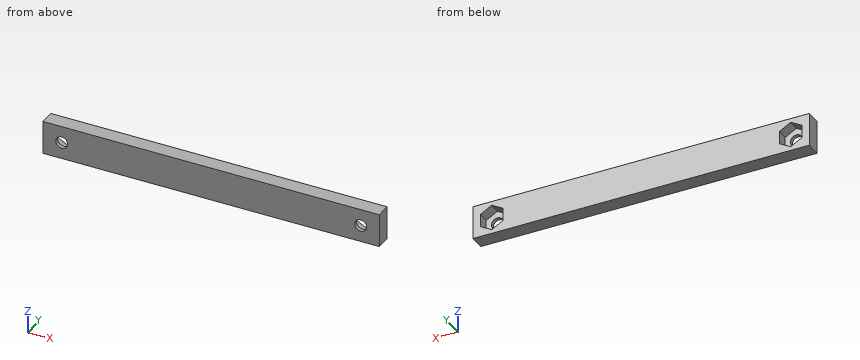
from build123d import *

# Parameters (mm, degrees)
SKETCH089_W     = 90
SKETCH089_H     = 9
SKETCH089_R     = 1.6
PAD034_DEPTH    = 4
POCKET055_DEPTH = 3


with BuildPart() as part:
    # Sketch089 → Pad034 (new body)
    with BuildSketch(Plane.XZ):
        with Locations((0, 34)):
            Rectangle(SKETCH089_W, SKETCH089_H)
        with Locations((-40, 34)):
            Circle(SKETCH089_R, mode=Mode.SUBTRACT)
        with Locations((40, 34)):
            Circle(SKETCH089_R, mode=Mode.SUBTRACT)
    extrude(amount=PAD034_DEPTH)

    # Sketch090 (on Face7 of Pad034) → Pocket055 (cut)
    with BuildSketch(Plane(origin=(0, 0, 0), x_dir=(1, 0, 0), z_dir=(0, 1, 0))):
        Polygon((-37, -32.267949), (-40, -30.535898), (-43, -32.267949), (-43, -35.732051), (-40, -37.464102), (-37, -35.732051), align=None)
    pocket055 = extrude(amount=-POCKET055_DEPTH, mode=Mode.SUBTRACT)

    # Mirrored005: Pocket055 across Sketch090 V_Axis
    add(pocket055.mirror(Plane.YZ), mode=Mode.SUBTRACT)


with BuildPart() as part_1:
    # Body012 placement: moved
    add(part.part.moved(Location((0, 19, 100))))


solid = part_1.part
The listing builds one solid part. Answer for the finished solid, in the listing's coordinates (mm). Coordinates: 2 decimals unless noted, no trailing zeros. Order: outer loops, then holes, each group sorted by start corner. A loop starts at its lowest first (then second) coordinate and runs counter-clockwise, first axis right, second up. Notation, with made-up numbers: (-29, -28) -> (-5, -28) arc R25 ccw to (-5, -13) -> close; hole circle Ø1 at (80.25, -24). An arc over 180 degrees is marked (long way). Answer in a Markdown table with one row per item. Add a question column.
Item 1: Find section A-A (y = 18.2). Write down the section's boundary in (x, z).
Item 2: Find section B-B (z = 134). Write down the section's boundary in (x, y).
Item 3: This flat-tipped pin is pushed along its axis until it touches: P1, Ø3.5, axis at x = 40, z = 134, coming from the +Y side. Where does it stop, or does it pass through?
Item 4: Find the intervals of material crossed by L1, parallel to X at y = 15.3, z = 134; L2, parallel to Z at x = 40, y = 15.7; L3, parallel to X at y = 16.65, z = 132.25, in increasing order. Write a range as from..to.
Result set:
| question | item | result |
|---|---|---|
| 1 | outline | (-45, 129.5) -> (45, 129.5) -> (45, 138.5) -> (-45, 138.5) -> close; hole (-43, 132.27) -> (-40, 130.54) -> (-37, 132.27) -> (-37, 135.73) -> (-40, 137.46) -> (-43, 135.73) -> close; hole (37, 132.27) -> (40, 130.54) -> (43, 132.27) -> (43, 135.73) -> (40, 137.46) -> (37, 135.73) -> close |
| 2 | outline | (-45, 15) -> (-41.6, 15) -> (-41.6, 16) -> (-43, 16) -> (-43, 19) -> (-45, 19) -> close; (-38.4, 15) -> (38.4, 15) -> (38.4, 16) -> (37, 16) -> (37, 19) -> (-37, 19) -> (-37, 16) -> (-38.4, 16) -> close; (41.6, 15) -> (45, 15) -> (45, 19) -> (43, 19) -> (43, 16) -> (41.6, 16) -> close |
| 3 | P1 | stops at y = 16 |
| 4 | L1 | x = -45..-41.6, -38.4..38.4, 41.6..45 |
| 4 | L2 | z = 129.5..132.4, 135.6..138.5 |
| 4 | L3 | x = -45..-42.97, -37.03..37.03, 42.97..45 |
